Here's the drawing with two shaded views (mm, measured from the low corner). I have some questions. Round coordinates to 2 decimals unless told otherwise and drop trailing zeros. Write each loop counter-clockwise with the first axis right and the second up, starting at its lowest first coordinate (ties: lowest second). Pieces come first, ordered by that corner, then holes. Notation, with made-up numbers: M 6.25,-10 L 18.25,-10 A20 cw 18.25,16 Z; hole C -18,5.5 d2. An arc over 180 degrees is marked long. Use one line per item in the form item = value. Start each with the question number.
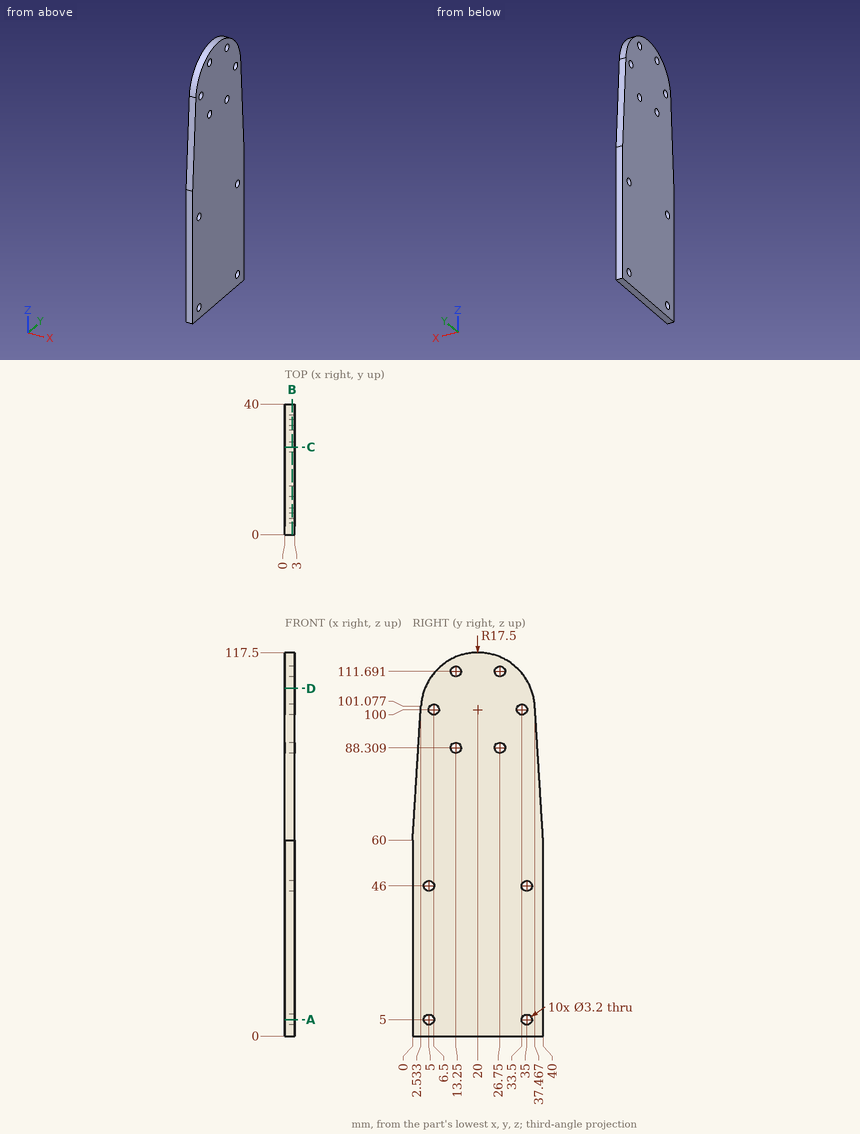
1. Will these pins go through, and if not, where does the flat tip stop? pin 1 (1 mm diameter, centred on x = 1.5, y = 15.5, fed in from +Z); pin 2 (1.5 mm diameter, centred on x = 1.5, z = 96.5, fed in from +Y) (1 decimal); pin 3 (1 mm diameter, centred on x = 1.5, y = 32.5, fed in from +Z).
2. Please list where these lines run through material, in increasing order: line 1 along Y through (x, z) = (1.25, 5); line 2 along Y through (x, z) = (0.85, 100); line 3 along Z through (x, y) = (1.25, 13.25) (1 decimal).
3. If we section it at A-A (z = 5): List the corners of the cut face in (x, y) for me, and give its area (3 significant figures).
4. If we section it at D-D (z = 106.5): List the corners of the cut face in (x, y) for me.
5. If we section it at B-B (x = 2.25): State how many separate pieces and enclosed holes the cut face has, and give its area (3 significant figures).
6. If we section it at C-C (y = 26.75): List the corners of the cut face in (x, z) for me.
Model answer:
q1.pin_1 = 117.04
q1.pin_2 = 37.8
q1.pin_3 = 112.74
q2.line_1 = 0 to 3.4, 6.6 to 33.4, 36.6 to 40
q2.line_2 = 2.47 to 4.9, 8.1 to 31.9, 35.1 to 37.53
q2.line_3 = 0 to 86.7, 89.9 to 110.1, 113.3 to 116.1
q3.outline = M 0,0 L 3,0 L 3,3.4 L 0,3.4 Z; M 0,6.6 L 3,6.6 L 3,33.4 L 0,33.4 Z; M 0,36.6 L 3,36.6 L 3,40 L 0,40 Z
q3.area = 101 mm2
q4.outline = M 0,3.75 L 3,3.75 L 3,36.25 L 0,36.25 Z
q5.separate_pieces = 1
q5.enclosed_holes = 10
q5.area = 4,300 mm2
q6.outline = M 0,0 L 3,0 L 3,86.71 L 0,86.71 Z; M 0,89.91 L 3,89.91 L 3,110.09 L 0,110.09 Z; M 0,113.29 L 3,113.29 L 3,116.15 L 0,116.15 Z
